```python
from build123d import *

# Parameters (mm, degrees)
F0_W     = 50.8
F0_H     = 50.8
F1_DEPTH = 50.8
F2_W     = 25.4
F2_H     = 25.4
F3_DEPTH = 12.7
F4_R     = 10.22151
F5_DEPTH = 25.4


with BuildPart() as f1:
    # F0 (on Front) → F1 (new body)
    with BuildSketch(Plane.XZ):
        with Locations((-25.4, 25.4)):
            Rectangle(F0_W, F0_H)
    extrude(amount=F1_DEPTH)

    # F2 (on face) → F3 (join)
    with BuildSketch(Plane(origin=(0, 0, 0), x_dir=(-1, 0, 0), z_dir=(0, 1, 0))):
        with Locations((26.126995, 28.438128)):
            Rectangle(F2_W, F2_H)
    extrude(amount=F3_DEPTH)

    # F4 (on face) → F5 (cut)
    with BuildSketch(Plane(origin=(0, 0, 0), x_dir=(1, 0, 0), z_dir=(0, 0, -1))):
        with Locations((-21.743661, 26.524765)):
            Circle(F4_R)
    extrude(amount=-F5_DEPTH, mode=Mode.SUBTRACT)


solid = f1.part
```
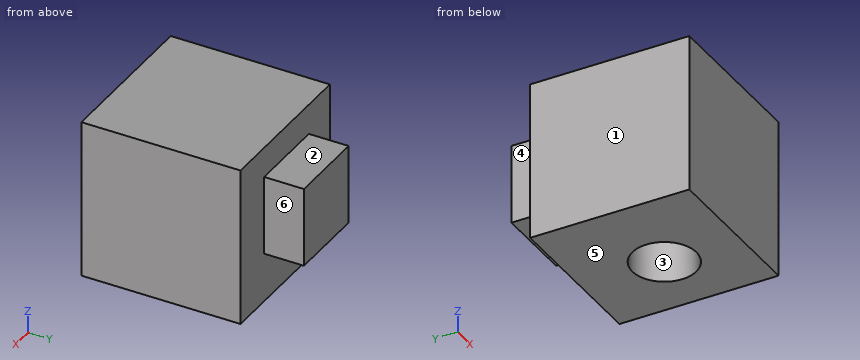
Model file for the job. Use its own axes, mm. Face numbers are marked on the shaded views. A direction names the side the tool comes from. Coordinates: 2 decimals unless noted, no trailing zeros. Order: outer loops, then holes, each group sorted by start corner. A loop starts at its lowest first (then second) coordinate and runs counter-clockwise, first axis right, second up. Notation, with made-up numbers: (-18, 72) - (-10, 72) arc R24 ccw to (-10, 99) - close; hole circle Ø9 at (52, 82.5). An arc over 180 degrees is marked (long way). Return JSON: item names as keys, results as strings. Group by question number.
1) Saw through at C-C, the plane z = 10.5. Write the cut outline in (x, y).
2) Mould opens along X. For the marked faces 3, 4, 5 and 6 say: released by +X, released by -X, zero draft, split by the parting line, or undercut.
3) Saw through at B-B, the plane y = -23. Write the cut outline in (x, z), plus the area to 3 significant figures.
4) Saw through at D-D, the plane y = 1.5. Write the cut outline in (x, z).
5) Probe line 1 (Y direction, x = -22, z = 20); line 2 (X direction, y = 5, z = 41); line 3 (Y direction, x = -46, z = 29). List the from-to ranges inside material, lowest first. Write a range as from..to.
6) Saw through at A-A, the plane x = -33.5. Write the cut outline in (y, z), plus the area to 3 significant figures.
7) Tool access for the marked faces 1 and 2: list every direction of +Z, -Z, +X, -X, +Y, -Y with a clear straight run to the whole face (end or side of a thin tool).
8) Flat gauge pins, fed straight in: P1, Ø6.5, axis at x = -27, y = 8, coming from the +Z side; P2, Ø10, axis at y = 6, z = 27.5, coming from the -X side; P3, Ø10, axis at x = -31.5, y = 6.5, coming from the -Z side. Where does each tip first touch, or does it go through?
Values found:
{
 "1": {"outline": "(-50.8, -50.8) - (0, -50.8) - (0, 0) - (-50.8, 0) - close; hole circle Ø20.44 at (-21.74, -26.52)"},
 "2": {"face 3": "undercut", "face 4": "released by -X", "face 5": "zero draft", "face 6": "released by +X"},
 "3": {"outline": "(-50.8, 0) - (-31.34, 0) - (-31.34, 25.4) - (-12.15, 25.4) - (-12.15, 0) - (0, 0) - (0, 50.8) - (-50.8, 50.8) - close", "area": "2,090 mm²"},
 "4": {"outline": "(-38.83, 15.74) - (-13.43, 15.74) - (-13.43, 41.14) - (-38.83, 41.14) - close"},
 "5": {"line 1": "y = -50.8..-36.74, -16.31..12.7", "line 2": "x = -38.83..-13.43", "line 3": "y = -50.8..0"},
 "6": {"outline": "(-50.8, 0) - (0, 0) - (0, 15.74) - (12.7, 15.74) - (12.7, 41.14) - (0, 41.14) - (0, 50.8) - (-50.8, 50.8) - close", "area": "2,900 mm²"},
 "7": {"face 1": "+Z, -Z, -X, +Y, -Y", "face 2": "+Z, +X, -X, +Y"},
 "8": {"P1": "stops at z = 41.14", "P2": "stops at x = -38.83", "P3": "stops at z = 15.74"}
}
